Source: CAD feature listing. Evaluate the final solid. Frame: model axes, mm. Face numbers are marked on the shaded views. A direction names the side the tool comes from. Coordinates: 2 decimals unless noted, no trailing zeros. Loops run counter-clockwise (first coordinate to the right, second up) from the corner with the lowest first, then second, coordinate; pieces in that order, holes last. Notation, with made-up numbers: (-26, -15) -> (22, -15) arc R25 ccw to (22, 17) -> close; hole circle Ø2 at (-12, 86). An arc over 180 degrees is marked (long way). Answer as a JSON object with one key per item and string values. Group by question number.
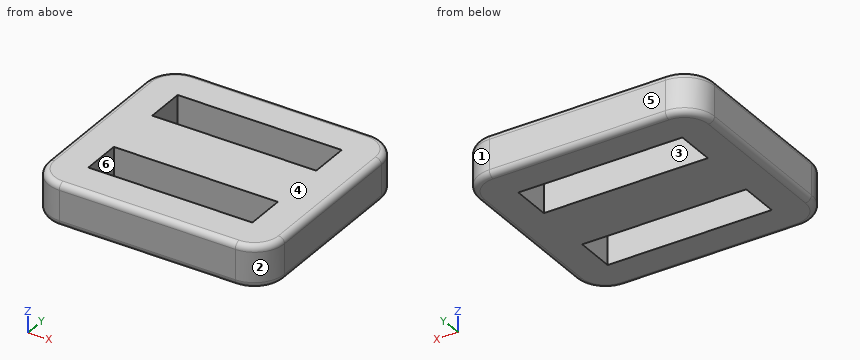
Autodesk Fusion 360 part; units mm, degrees
sketch "Sketch1" plane through (0, 0, 0) normal (0, 0, 1) x (1, 0, 0)
  line L0 (32.604, 29.4843) -> (52.304, 29.4843)
  line L1 (52.304, 29.4843) -> (52.304, 11.8843)
  line L2 (52.304, 11.8843) -> (32.604, 11.8843)
  line L3 (32.604, 11.8843) -> (32.604, 29.4843)
  line L4 (35.604, 26.4843) -> (49.304, 26.4843)
  line L5 (49.304, 26.4843) -> (49.304, 23.1843)
  line L6 (49.304, 23.1843) -> (35.604, 23.1843)
  line L7 (35.604, 23.1843) -> (35.604, 26.4843)
  line L8 (35.604, 18.1843) -> (49.304, 18.1843)
  line L9 (49.304, 18.1843) -> (49.304, 14.8843)
  line L10 (49.304, 14.8843) -> (35.604, 14.8843)
  line L11 (35.604, 14.8843) -> (35.604, 18.1843)
  dimension "d2" = 3.3
  dimension "d3" = 3.3
  dimension "d4" = 13.7
  dimension "d5" = 13.7
  dimension "d6" = 5
  dimension "d7" = 3
  dimension "d8" = 3
  dimension "d9" = 3
  dimension "d10" = 3
  dimension "d11" = 3
extrude "Extrude1" add sketch "Sketch1" along normal blind 3.5
fillet "Fillet1" radius 2.5 4 edges at (32.604, 29.4843, 1.75) (52.304, 29.4843, 1.75) (32.604, 11.8843, 1.75) (52.304, 11.8843, 1.75)
fillet "Fillet2" radius 0.5 16 edges at (51.5717, 12.6165, 3.5) (52.304, 20.6843, 3.5) (51.5717, 28.752, 3.5) (42.454, 29.4843, 3.5) (33.3362, 28.752, 3.5) (32.604, 20.6843, 3.5) (33.3362, 12.6165, 3.5) (42.454, 11.8843, 3.5) (33.3362, 12.6165, 0) (32.604, 20.6843, 0) (33.3362, 28.752, 0) (42.454, 29.4843, 0) (51.5717, 28.752, 0) (52.304, 20.6843, 0) (51.5717, 12.6165, 0) (42.454, 11.8843, 0)
equation "d3 = 3 mm + 0.3 mm"
equation "d4 = 0.5 in + 1 mm"
equation "d5 = 0.5 in + 1 mm"
1. Mould query, pull axis Y, two halves, no side actions, for the marked faces 1, 2, 3 and 4. Classes: pulls with the +Y half, pulls with the -Y half, needs draft (parallel to the pull), parting line crosses it, or undercut.
2. Ray query, L1, parallel to Y at x = 39, z = 2.2; L2, parallel to X at y = 25.5, z = 0.45; L3, parallel to X at y = 24, z = 3.35. Return the intervals inside material, ascending.
3. Reachability of the marked faces 5 and 6 from +Z, -Z, +X, -X, +Y, -Y: full face, straight path, thin tool, end or side. Return the list, or none.
4. Section query D-D on z = 3.25. Return loops of the section in (x, y), then the cut area to 3 significant figures.
5. Section query B-B on y = 17.5. Return loops of the section in (x, z).
6. Section query A-A on x = 38.75. Return loops of the section in (y, z).
7. Section query C-C on z = 2. Return loops of the section in (x, y), then the cut area to 3 significant figures.
Solved:
{
 "1": {"face 1": "pulls with the +Y half", "face 2": "pulls with the -Y half", "face 3": "undercut", "face 4": "needs draft"},
 "2": {"L1": "11.88 to 14.88, 18.18 to 23.18, 26.48 to 29.48", "L2": "32.61 to 35.6, 49.3 to 52.3", "L3": "32.75 to 35.6, 49.3 to 52.16"},
 "3": {"face 5": "+Z, -Z, +X, -X, +Y", "face 6": "+Z, -Z"},
 "4": {"outline": "(32.67, 14.38) arc R2.43 ccw to (35.1, 11.95) -> (49.8, 11.95) arc R2.43 ccw to (52.24, 14.38) -> (52.24, 26.98) arc R2.43 ccw to (49.8, 29.42) -> (35.1, 29.42) arc R2.43 ccw to (32.67, 26.98) -> close; hole (35.6, 14.88) -> (49.3, 14.88) -> (49.3, 18.18) -> (35.6, 18.18) -> close; hole (35.6, 23.18) -> (49.3, 23.18) -> (49.3, 26.48) -> (35.6, 26.48) -> close", "area": "246 mm^2"},
 "5": {"outline": "(32.6, 0.5) arc R0.5 ccw to (33.1, 0) -> (35.6, 0) -> (35.6, 3.5) -> (33.1, 3.5) arc R0.5 ccw to (32.6, 3) -> close; (49.3, 0) -> (51.8, 0) arc R0.5 ccw to (52.3, 0.5) -> (52.3, 3) arc R0.5 ccw to (51.8, 3.5) -> (49.3, 3.5) -> close"},
 "6": {"outline": "(11.88, 0.5) arc R0.5 ccw to (12.38, 0) -> (14.88, 0) -> (14.88, 3.5) -> (12.38, 3.5) arc R0.5 ccw to (11.88, 3) -> close; (18.18, 0) -> (23.18, 0) -> (23.18, 3.5) -> (18.18, 3.5) -> close; (26.48, 0) -> (28.98, 0) arc R0.5 ccw to (29.48, 0.5) -> (29.48, 3) arc R0.5 ccw to (28.98, 3.5) -> (26.48, 3.5) -> close"},
 "7": {"outline": "(32.6, 14.38) arc R2.5 ccw to (35.1, 11.88) -> (49.8, 11.88) arc R2.5 ccw to (52.3, 14.38) -> (52.3, 26.98) arc R2.5 ccw to (49.8, 29.48) -> (35.1, 29.48) arc R2.5 ccw to (32.6, 26.98) -> close; hole (35.6, 14.88) -> (49.3, 14.88) -> (49.3, 18.18) -> (35.6, 18.18) -> close; hole (35.6, 23.18) -> (49.3, 23.18) -> (49.3, 26.48) -> (35.6, 26.48) -> close", "area": "251 mm^2"}
}
